Autodesk Inventor part; units mm, degrees
ref_plane "YZ Plane" through (0, 0, 0) normal (1, 0, 0) x (0, 1, 0)
ref_plane "XZ Plane" through (0, 0, 0) normal (0, 1, 0) x (-1, 0, 0)
ref_plane "XY Plane" through (0, 0, 0) normal (0, 0, 1) x (1, 0, 0)
sketch "Sketch1" plane through (0, 0, 0) normal (0, 1, 0) x (-1, 0, 0)
  line L0 (0, 0) -> (0, -16)
  line L1 (0, -16) -> (4, -16)
  line L2 (0, 0) -> (4, 0)
  line L3 (4, 0) -> (4, -6)
  line L4 (4, -16) -> (4, -13)
  line L5 (4, -13) -> (7, -13)
  line L6 (7, -13) -> (7, -4)
  line L7 (7, -4) -> (4, -6)
  dimension "d0" = 16
  dimension "d1" = 4
  dimension "d2" = 6
  dimension "d3" = 3
  dimension "d4" = 3
  dimension "d5" = 9
extrude "Extrusion1" add sketch "Sketch1" along normal blind 32
sketch "Sketch2" plane through (-7, 0, -13) normal (-1, 0, 0) x (0, 0, 1)
  line L0 (0, 0) -> (9, 0)
  line L1 (9, 0) -> (9, 32)
  line L2 (0, 32) -> (9, 32)
  line L3 (0, 0) -> (0, 32)
  line L4 (0, 0) -> (9, 0)
  line L5 (5.5, 0) -> (5.5, 25)
  line L6 (5.5, 25) -> (0, 25)
  point P0 (13, 0)
  dimension "d8" = 25
  dimension "d9" = 5.5
extrude "Extrusion2" cut sketch "Sketch2" against normal blind 3 contours L3 L6 L5 L0
sketch "Sketch3" plane through (-4, 0, -16) normal (-1, 0, 0) x (0, 0, 1)
  line L0 (0, 0) -> (8.5, 0)
  line L1 (8.5, 25) -> (8.5, 0)
  line L2 (3, 25) -> (8.5, 25)
  line L3 (3, 25) -> (3, 32)
  line L4 (0, 32) -> (3, 32)
  line L5 (0, 0) -> (0, 32)
  line L6 (0, 0) -> (8.5, 0)
  line L7 (0, 0) -> (0, 12)
  line L8 (0, 0) -> (0, 32)
  line L9 (0, 12) -> (3, 12)
  line L10 (3, 12) -> (3, 15)
  line L11 (3, 15) -> (8.5, 15)
  line L12 (8.5, 25) -> (8.5, 0)
  line L13 (3, 25) -> (3, 32)
  line L14 (3, 25) -> (0, 25)
  point P0 (16, 0)
  dimension "d12" = 12
  dimension "d13" = 3
  dimension "d14" = 3
extrude "Extrusion3" cut sketch "Sketch3" against normal blind 4 contours L5 L14 L2 L1 L11 L10 L9
properties part number "Inner Rails 2"
Design review of the part built by this model. Coordinates are the model's own, in mm. A direction names the side the tool comes from. Coordinates: 2 decimals unless noted, no trailing zeros. Order: outer loops, then holes, each group sorted by start corner. A loop starts at its lowest first (then second) coordinate and runs counter-clockwise, first axis right, second up. Notation, with made-up numbers: (17, 80.25) - (38, 80.25) arc R19 cw to (38, 116.25) - close; hole circle Ø2 at (-38.75, -5.5). An arc over 180 degrees is marked (long way). Answer in a Markdown table with one row per item.
(1) Clearance check with flat-ended pins moving along their axes: pin 1 (2.5 mm diameter, centred on y = 29.5, z = -14.5, fed in from -X); pin 2 (0.9 mm diameter, centred on x = -1.5, y = 13.5, fed in from -Z); pin 3 (2 mm diameter, centred on x = -6.5, y = 12.5, fed in from -Z). State where each tip first meets the part, or that it passes through.
Checked values:
| item | result |
|---|---|
| pin 1 | x = -4 |
| pin 2 | z = -13 |
| pin 3 | z = -7.5 |
(2) Consider section B-B on y = 27. State the section outline as (x, z) points.
Checked values:
| item | result |
|---|---|
| outline | (-7, -13) - (-4, -13) - (-4, -16) - (0, -16) - (0, 0) - (-4, 0) - (-4, -6) - (-7, -4) - close |
(3) Wall thickness on line 1 along Y through (x, z) = (-1.75, -12); line 2 along Y through (x, z) = (-4.75, -11.75); line 3 along X through (y, z) = (2, -9.25): over which ranges is each line inside the solid? List them lowest first. Write a range as from..to.
Checked values:
| item | result |
|---|---|
| line 1 | 0..15, 25..32 |
| line 2 | 25..32 |
| line 3 | -4..0 |
(4) Consider section C-C on x = -1.75. State the section outline as (y, z) points, plus the area to 3 significant figures.
Checked values:
| item | result |
|---|---|
| outline | (0, -16) - (12, -16) - (12, -13) - (15, -13) - (15, -7.5) - (25, -7.5) - (25, -16) - (32, -16) - (32, 0) - (0, 0) - close |
| area | 418 mm^2 |
(5) The part is to be moulded in two halves that separate along Y. For faces 4 (the flat face through (-2, 0, -8)), 5 (the flat face through (-5, 28, -13)), 6 (the flat face through (-3, 32, -8)), 7 (the flat face through (-2, 12, -15)), say which applies: released by +Y, released by -Y, zero draft, split by the parting line, or undercut.
Checked values:
| item | result |
|---|---|
| face 4 | released by -Y |
| face 5 | zero draft |
| face 6 | released by +Y |
| face 7 | undercut |
(6) Consider section A-A on z = -8.5. State the section outline as (x, y) points, plus the area to 3 significant figures.
Checked values:
| item | result |
|---|---|
| outline | (-7, 25) - (0, 25) - (0, 32) - (-7, 32) - close; (-4, 0) - (0, 0) - (0, 15) - (-4, 15) - close |
| area | 109 mm^2 |
(7) Consider section D-D on z = -13.75. State the section outline as (x, y) points.
Checked values:
| item | result |
|---|---|
| outline | (-4, 0) - (0, 0) - (0, 12) - (-4, 12) - close; (-4, 25) - (0, 25) - (0, 32) - (-4, 32) - close |
(8) For faces 1 (the flat face through (-4, 25, -11)), 2 (the flat face through (-4, 29, -15)), 3 (the flat face through (-5.5, 15.8, -5)), list the 3-axis set-ups (+Z, -Z, +X, -X, +Y, -Y) from which the entire face can be reached by the end or side of a thin tool; tool diameter is ignored.
Checked values:
| item | result |
|---|---|
| face 1 | -Z, +X, -X |
| face 2 | -Z, -X, +Y, -Y |
| face 3 | +Z, +Y, -Y |
